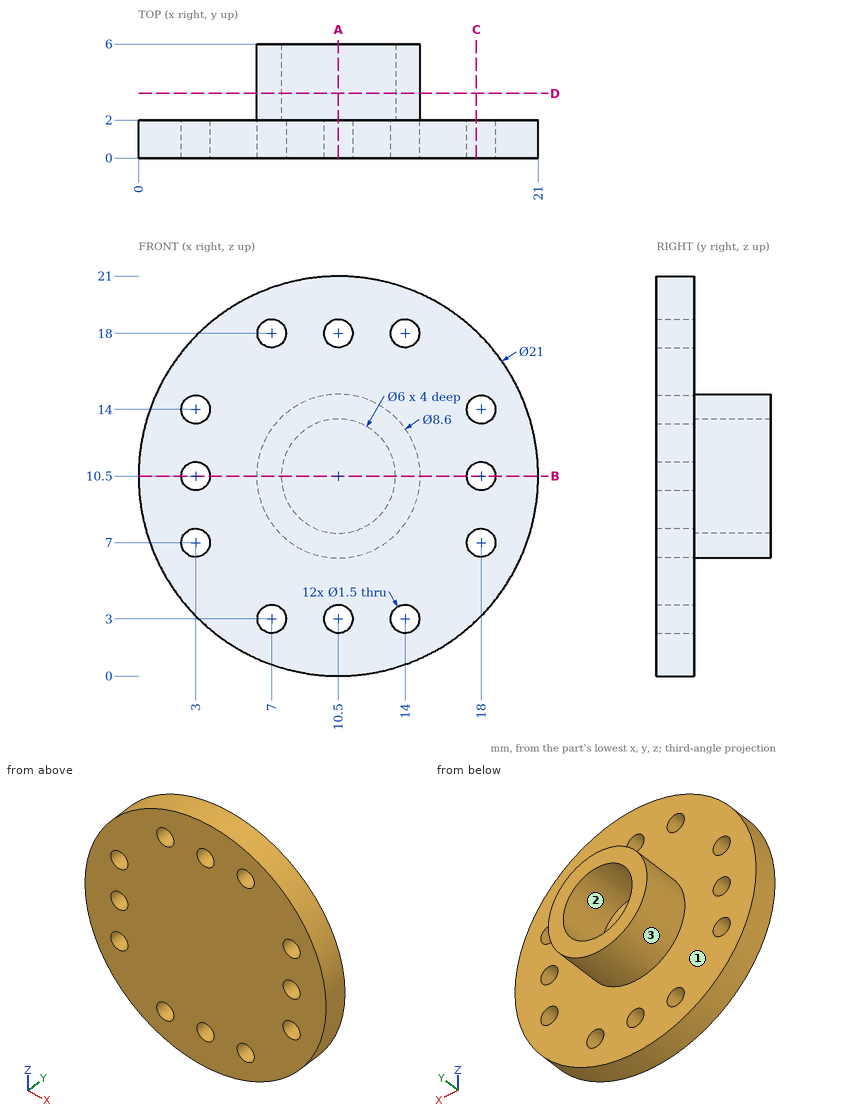
Can you work these out from the drawing? Everything is in mm from the part's minimum corner. Round coordinates to 2 decimals unless told otherwise and drop trailing zeros. Order: outer loops, then holes, each group sorted by start corner. A loop starts at its lowest first (then second) coordinate and runs counter-clockwise, first axis right, second up. Notation, with made-up numbers: (-10.5, 40) - (13.5, 40) arc R34 ccw to (13.5, 79) - close; hole circle Ø10 at (12.25, -9.5). An arc over 180 degrees is marked (long way). Answer in a Markdown table with one row per item.
(1) Suppose I cut it at B-B, the plane z = 10.5. Please give me the cut outline in (x, y), plus the area to 3 significant figures.
From the geometry:
| item | result |
|---|---|
| outline | (0, 0) - (2.25, 0) - (2.25, 2) - (0, 2) - close; (3.75, 0) - (17.25, 0) - (17.25, 2) - (14.8, 2) - (14.8, 6) - (13.5, 6) - (13.5, 2) - (7.5, 2) - (7.5, 6) - (6.2, 6) - (6.2, 2) - (3.75, 2) - close; (18.75, 0) - (21, 0) - (21, 2) - (18.75, 2) - close |
| area | 46.4 mm2 |
(2) If we mould it in two halves opening along Z, with no side actions, what happens to the marked faces 1, 2 and 3? For each: released by +Z, released by -Z, zero draft, split by the parting line, or undercut.
From the geometry:
| item | result |
|---|---|
| face 1 | zero draft |
| face 2 | undercut |
| face 3 | split by the parting line |
(3) For P1, Ø1.7, axis at x = 7, z = 3, coming from the +Y side; P2, Ø2, axis at y = 5, z = 7.5, coming from the -X side, each with a flat end and sliding along its axis, tell me the tip position at first contact or that it passes through.
From the geometry:
| item | result |
|---|---|
| P1 | stops at y = 2 |
| P2 | stops at x = 6.69 |
(4) Please list where these lines run through material, in increasing order: L1, parallel to X at y = 1.95, z = 17.5; L2, parallel to Z at x = 10.5, y = 0.95; L3, parallel to X at y = 0.6, z = 18. Write a range as from..to.
From the geometry:
| item | result |
|---|---|
| L1 | x = 2.67..6.44, 7.56..9.94, 11.06..13.44, 14.56..18.33 |
| L2 | z = 0..2.25, 3.75..17.25, 18.75..21 |
| L3 | x = 3.15..6.25, 7.75..9.75, 11.25..13.25, 14.75..17.85 |
(5) Suppose I cut it at A-A, the plane x = 10.5. Please give me the cut outline in (y, z).
From the geometry:
| item | result |
|---|---|
| outline | (0, 0) - (2, 0) - (2, 2.25) - (0, 2.25) - close; (0, 3.75) - (2, 3.75) - (2, 6.2) - (6, 6.2) - (6, 7.5) - (2, 7.5) - (2, 13.5) - (6, 13.5) - (6, 14.8) - (2, 14.8) - (2, 17.25) - (0, 17.25) - close; (0, 18.75) - (2, 18.75) - (2, 21) - (0, 21) - close |
(6) Suppose I cut it at C-C, the plane x = 17.75. Please give me the cut outline in (y, z), plus the area to 3 significant figures.
From the geometry:
| item | result |
|---|---|
| outline | (0, 2.9) - (2, 2.9) - (2, 6.29) - (0, 6.29) - close; (0, 7.71) - (2, 7.71) - (2, 9.79) - (0, 9.79) - close; (0, 11.21) - (2, 11.21) - (2, 13.29) - (0, 13.29) - close; (0, 14.71) - (2, 14.71) - (2, 18.1) - (0, 18.1) - close |
| area | 21.9 mm2 |
(7) Suppose I cut it at D-D, the plane y = 3.4. Please give me the cut outline in (x, z).
From the geometry:
| item | result |
|---|---|
| outline | circle Ø8.6 at (10.5, 10.5); hole circle Ø6 at (10.5, 10.5) |
